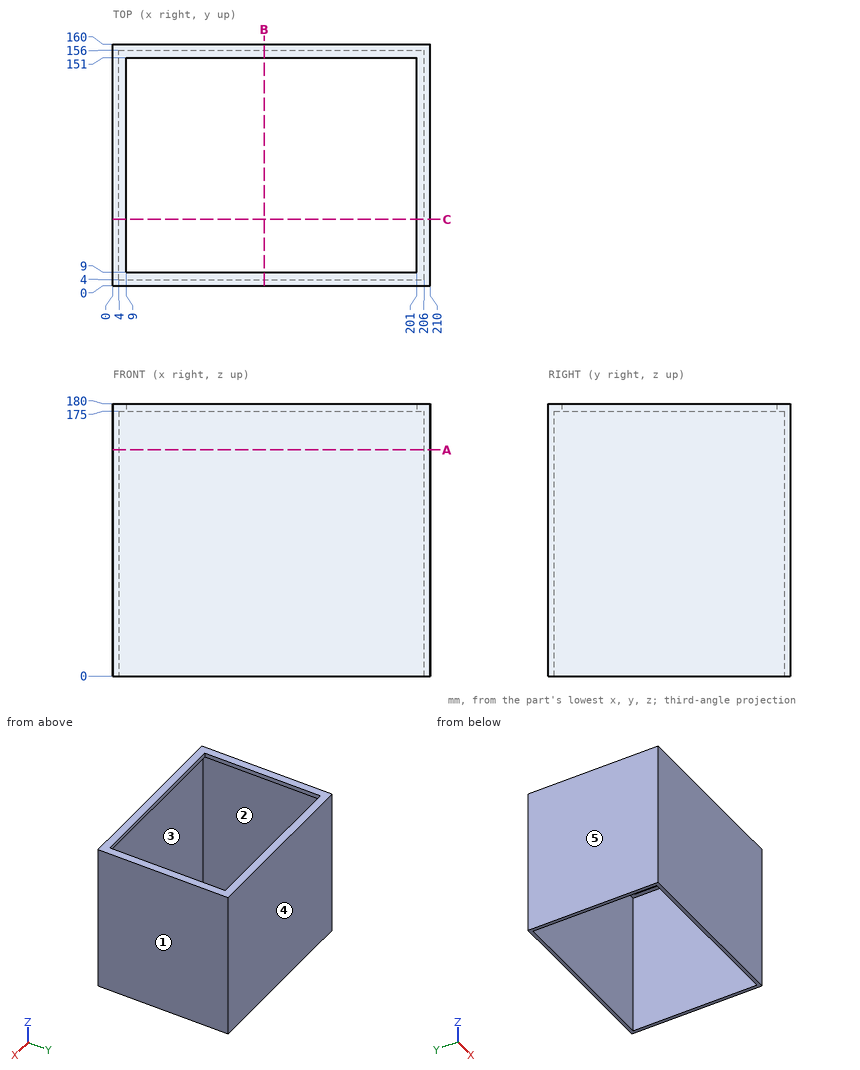
Here's the drawing with two shaded views (mm, measured from the low corner). I have some questions. A direction names the side the tool comes from. Give positions to 0.01 mm unless a question says otherwise; leave off trailing zeros. Order: outer loops, then holes, each group sorted by start corner. A loop starts at its lowest first (then second) coordinate and runs counter-clockwise, first axis right, second up. Notation, with made-up numbers: (85, 15) - (142, 15) arc R30 ccw to (142, 46) - close; hole circle Ø1 at (-31, 17). An arc over 180 degrees is marked (long way). Use a Markdown table: item, result. Add a question column.
Q1. If we mould it in two halves opening along X, with no side actions, what happens to the marked faces 3, 4 and 5? For each: released by +X, released by -X, zero draft, split by the parting line, or undercut.
Q2. If we section it at C-C on y = 44: Write out the boundary of the cut face in (x, z).
Q3. If we section it at A-A on z = 149.5: Write out the boundary of the cut face in (x, y), plus the area to 3 significant figures.
Q4. Please list where these lines run through material, in increasing order: line 1 along Y through (x, z) = (37, 117.5); line 2 along X through (y, z) = (130, 109).
Q5. I'm going to push a flat-ended pin straight in: pin 1 (4 mm diameter, centred on y = 48, z = 178, fed in from -X). Where does the tip first touch, or does it pass through?
Q6. On a 3-axis mill with a long thin cutter (end or side, diameter ignored), from which of +Z, -Z, +X, -X, +Y, -Y can I reach the whole of each face in a straight line? I mean the marked faces 1 and 2. Say none if no direction works.
Q7. If we section it at B-B on x = 100: Write out the boundary of the cut face in (y, z), plus the area to 3 significant figures.
Answers follow:
| question | item | result |
|---|---|---|
| 1 | face 3 | undercut |
| 1 | face 4 | zero draft |
| 1 | face 5 | released by -X |
| 2 | outline | (0, 0) - (4, 0) - (4, 175) - (9, 175) - (9, 180) - (0, 180) - close; (201, 175) - (206, 175) - (206, 0) - (210, 0) - (210, 180) - (201, 180) - close |
| 3 | outline | (0, 0) - (210, 0) - (210, 160) - (0, 160) - close; hole (4, 4) - (206, 4) - (206, 156) - (4, 156) - close |
| 3 | area | 2,900 mm^2 |
| 4 | line 1 | y = 0 to 4, 156 to 160 |
| 4 | line 2 | x = 0 to 4, 206 to 210 |
| 5 | pin 1 | stops at x = 0 |
| 6 | face 1 | +Z, -Z, +X, +Y, -Y |
| 6 | face 2 | -Z |
| 7 | outline | (0, 0) - (4, 0) - (4, 175) - (9, 175) - (9, 180) - (0, 180) - close; (151, 175) - (156, 175) - (156, 0) - (160, 0) - (160, 180) - (151, 180) - close |
| 7 | area | 1,490 mm^2 |
